from build123d import *

# Parameters (mm, degrees)
SKETCH2_R = 0.25


with BuildPart() as part:
    # Sweep1: sweep along a path in Sketch1
    with BuildLine(Plane.XY) as sweep1_path:
        Line((-5.08, -3.4), (-5.08, -0.75))
        ThreePointArc((-5.08, -0.75), (-4.860330086, -0.219669914), (-4.33, 0))
        Line((-4.33, 0), (4.33, 0))
        ThreePointArc((4.33, 0), (4.860330086, -0.219669914), (5.08, -0.75))
        Line((5.08, -0.75), (5.08, -3.4))
    # Sketch2 → Sweep1 (sweep)
    with BuildSketch(Plane(origin=(-5.08, -3.4, 0), x_dir=(-1, 0, 0), z_dir=(0, -1, 0))):
        Circle(SKETCH2_R)
    sweep(path=sweep1_path.line)

    # Sketch3 → Revolve1 (revolve)
    with BuildSketch(Plane.XY, mode=Mode.PRIVATE) as revolve1_sk:
        with BuildLine():
            Line((-3, 0.25), (-3, 0))
            Line((-3, 0), (3, 0))
            Line((3, 0), (3, 0.25))
            ThreePointArc((3, 0.25), (2.733467171, 0.893467171), (2.09, 1.16))
            ThreePointArc((2.09, 1.16), (1.710392802, 1.117024996), (1.35, 0.990275229))
            ThreePointArc((1.35, 0.990275229), (1.179543945, 0.930326015), (1, 0.91))
            Line((1, 0.91), (-1, 0.91))
            ThreePointArc((-1, 0.91), (-1.179543945, 0.930326015), (-1.35, 0.990275229))
            ThreePointArc((-1.35, 0.990275229), (-1.710392802, 1.117024996), (-2.09, 1.16))
            ThreePointArc((-2.09, 1.16), (-2.733467171, 0.893467171), (-3, 0.25))
        make_face()
    revolve(revolve1_sk.sketch.rotate(Axis((-3, 0, 0), (1, 0, 0)), 90), axis=Axis((-3, 0, 0), (1, 0, 0)))

    # Sketch5 → Revolve2 (revolve)
    with BuildSketch(Plane.XY, mode=Mode.PRIVATE) as revolve2_sk:
        with BuildLine():
            ThreePointArc((2.09, 1.16), (1.864572551, 1.14822478), (1.643967886, 1.100373215))
            ThreePointArc((1.643967886, 1.100373215), (1.865, 1.145027293), (2.09, 1.16))
        make_face()
        with BuildLine():
            ThreePointArc((0.722381779, 0.91), (0.497381779, 0.915065065), (0.272381779, 0.91))
            Line((0.272381779, 0.91), (0.722381779, 0.91))
        make_face()
        with BuildLine():
            ThreePointArc((-0.138809111, 0.91), (-0.363809111, 0.915065065), (-0.588809111, 0.91))
            Line((-0.588809111, 0.91), (-0.138809111, 0.91))
        make_face()
        with BuildLine():
            ThreePointArc((-2.09, 1.16), (-1.959569758, 1.154983337), (-1.829910188, 1.139962988))
            ThreePointArc((-1.829910188, 1.139962988), (-2.054910188, 1.165604225), (-2.279910188, 1.139962988))
            ThreePointArc((-2.279910188, 1.139962988), (-2.185482147, 1.154976883), (-2.09, 1.16))
        make_face()
        with BuildLine():
            ThreePointArc((-1.35, 0.990275229), (-1.179543945, 0.930326015), (-1, 0.91))
            ThreePointArc((-1, 0.91), (-1.179019479, 0.931459747), (-1.34789488, 0.994622978))
            ThreePointArc((-1.34789488, 0.994622978), (-1.390151551, 1.013716419), (-1.434186266, 1.028246719))
            ThreePointArc((-1.434186266, 1.028246719), (-1.391834938, 1.009833416), (-1.35, 0.990275229))
        make_face()
    revolve(revolve2_sk.sketch.rotate(Axis((-3, 0, 0), (1, 0, 0)), 90), axis=Axis((-3, 0, 0), (1, 0, 0)))


solid = part.part
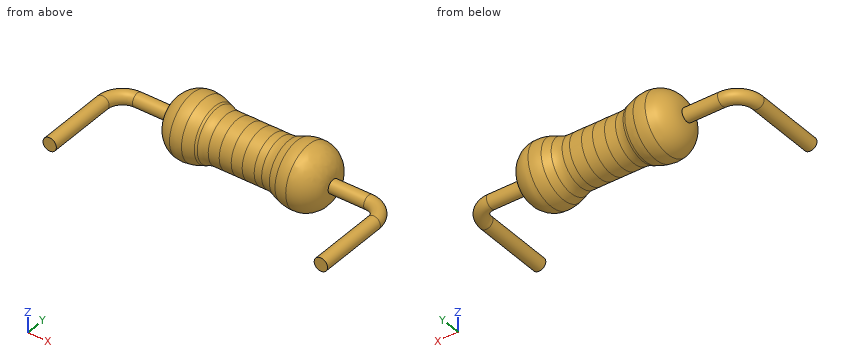
Verification items for the finished model (mm, model axes). Coordinates: 2 decimals unless noted, no trailing zeros. Order: outer loops, then holes, each group sorted by start corner. A loop starts at its lowest first (then second) coordinate and runs counter-clockwise, first axis right, second up. Notation, with made-up numbers: (-24.75, -31) -> (-10.75, -31) arc R26 ccw to (-10.75, -3) -> close; hole circle Ø1 at (44.5, -18). An arc over 180 degrees is marked (long way). Use CSV: the item, a comma, the result in double quotes. Start each with the question number.
Q1. Thickness scan on line 1 along Y through (x, z) = (1.5, -0.35); line 2 along Z through (x, y) = (-5, -2.55); line 3 along Y through (x, z) = (0.25, -0.7). Record the ranges inside material, lowest first.
Q2. Section check A-A, the plane y = -1.45. Record the cut outline in (x, z).
Q3. Section check B-B, the plane y = -0.6. Give the number of separate pieces and of enclosed holes in the cut face, and give its area (3 significant figures).
Returned:
1,line 1,"y = -0.99 to 0.99"
1,line 2,"z = -0.24 to 0.24"
1,line 3,"y = -0.58 to 0.58"
2,outline,"circle Ø0.5 at (-5.08, 0); circle Ø0.5 at (5.08, 0)"
3,separate pieces,"3"
3,enclosed holes,"0"
3,area,"9.57 mm^2"
